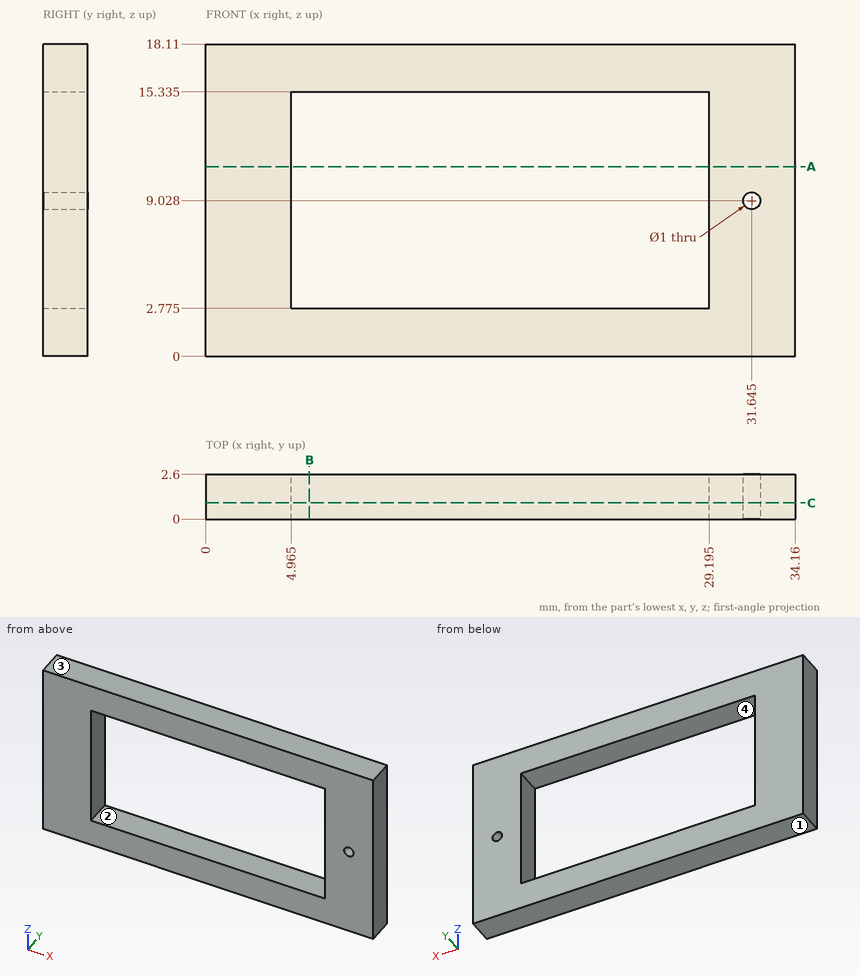
Verification items for this drawing (mm, ordinates from the low corner). A direction names the side the tool comes from. Round coordinates to 2 decimals unless told otherwise and drop trailing zeros. Loops run counter-clockwise (first coordinate to the right, second up) from the corner with the lowest first, then second, coordinate; pieces in that order, holes last. Notation, with made-up numbers: (13, 69) -> (28, 69) arc R16 cw to (28, 93) -> close; hole circle Ø4 at (-0.75, 82.5). An arc over 180 degrees is marked (long way). Answer in a Markdown table with one row per item.
Q1. Release check for a two-part mould opening along X. For the marked faces 3 and 4 record: released by +X, released by -X, zero draft, split by the parting line, or undercut.
Data:
| item | result |
|---|---|
| face 3 | zero draft |
| face 4 | undercut |
Q2. Thickness scan on L1, parallel to Z at x = 8, y = 1.2 (3 decimals); L2, parallel to X at y = 0.9, z = 11 (3 decimals); L3, parallel to X at y = 0.55, z = 9.25 (3 decimals). Record the ranges inside material, lowest first.
Data:
| item | result |
|---|---|
| L1 | z = 0 to 2.775, 15.335 to 18.11 |
| L2 | x = 0 to 4.965, 29.195 to 34.16 |
| L3 | x = 0 to 4.965, 29.195 to 31.197, 32.093 to 34.16 |
Q3. Sectioned sample at A-A on z = 11. Enter the section's corners in (x, y) (3 decimals), then the cut area to 3 significant figures.
Data:
| item | result |
|---|---|
| outline | (0, 0) -> (4.965, 0) -> (4.965, 2.6) -> (0, 2.6) -> close; (29.195, 0) -> (34.16, 0) -> (34.16, 2.6) -> (29.195, 2.6) -> close |
| area | 25.8 mm^2 |
Q4. Set-up check for the marked faces 1 and 2: record each of +Z, -Z, +X, -X, +Y, -Y from which the full face is reachable in a straight line by a thin tool's end or side.
Data:
| item | result |
|---|---|
| face 1 | -Z, +X, -X, +Y, -Y |
| face 2 | +Y, -Y |
Q5. Sectioned sample at C-C on y = 0.95. Enter the section's corners in (x, z) (3 decimals), then the cut area to 3 significant figures.
Data:
| item | result |
|---|---|
| outline | (0, 0) -> (34.16, 0) -> (34.16, 18.11) -> (0, 18.11) -> close; hole (4.965, 2.775) -> (29.195, 2.775) -> (29.195, 15.335) -> (4.965, 15.335) -> close; hole circle Ø1 at (31.645, 9.028) |
| area | 314 mm^2 |
Q6. Sectioned sample at B-B on x = 6. Enter the section's corners in (y, z) (3 decimals).
Data:
| item | result |
|---|---|
| outline | (0, 0) -> (2.6, 0) -> (2.6, 2.775) -> (0, 2.775) -> close; (0, 15.335) -> (2.6, 15.335) -> (2.6, 18.11) -> (0, 18.11) -> close |
